Geometry check sheet. Reference: the model listing, model coordinates, mm. Face numbers are marked on the shaded views. Coordinates: 2 decimals unless noted, no trailing zeros. Loops run counter-clockwise (first coordinate to the right, second up) from the corner with the lowest first, then second, coordinate; pieces in that order, holes last. Notation, with made-up numbers: (-33.75, 7.5) - (19.25, 7.5) arc R24 ccw to (19.25, 19.5) - close; hole circle Ø7 at (18, 33). An arc over 180 degrees is marked (long way). Write each question's results on one line, items separated by ' | '. Start each with the question number.
(1) Material ranges on probe 1 along X at (y, z) = (-23, 14.5); probe 2 along Y at (x, z) = (5, 4.75); probe 3 along X at (y, z) = (-15.5, 5), recorded low to high.
(2) Sectioned sample at C-C (x = 5). Enter the section's corners in (y, z), plus the area to 3 significant figures.
(3) Sectioned sample at A-A (x = 0). Enter the section's corners in (y, z).
(4) Sectioned sample at B-B (y = -33). Enter the section's corners in (x, z), plus the area to 3 significant figures.
(5) Go/stop test with flat-tipped pins: pin 1 Ø5 at (x, z) = (11.5, 4.5) entering from -Y; pin 2 Ø5 at (y, z) = (-3.5, 8.5) entering from -X; pin 3 Ø10 at (y, z) = (-1, 16.5) entering from +X; pin 4 Ø8 at (y, z) = (-27, 15.5) entering from -X. Record where each tip stops, or that it passes through.
(6) Mould release check, pull along Y, two halves, no side actions. Record for the marked faces 1 and 2: pulls with the +Y half, pulls with the -Y half, needs draft (parallel to the pull), parting line crosses it, or undercut.
from build123d import *

# Parameters (mm, degrees)
F1_DEPTH = 20
F2_R     = 1.59999


# Not quite as in the source:
# - a fillet or chamfer is up to 0.001 mm smaller than in the source, because OpenCascade refuses the exact size


with BuildPart() as f1:
    # F0 (on Top) → F1 (new body)
    with BuildSketch(Plane.XY):
        with BuildLine():
            ThreePointArc((6.05, 0), (5.4927369002, -2.5362060928), (3.9236061669, -4.6051943115))
            Line((3.9236061669, -4.6051943115), (-1.4025425598, -9.1430506051))
            ThreePointArc((-1.4025425598, -9.1430506051), (-0.799716174, -9.2153651062), (-0.1934443699, -9.2479770369))
            ThreePointArc((-0.1934443699, -9.2479770369), (1.8772842283, -8.6355074503), (4.015398341, -8.3330112302))
            ThreePointArc((4.015398341, -8.3330112302), (5.0486509404, -7.7507176237), (5.9989019907, -7.0409995672))
            ThreePointArc((5.9989019907, -7.0409995672), (8.3979861697, -3.8776704725), (9.25, 0))
            ThreePointArc((9.25, 0), (-1.6062456434, 9.1094717154), (-8.6921567423, -3.1636863258))
            Line((-8.6921567423, -3.1636863258), (-5.6851403558, -2.0692218671))
            ThreePointArc((-5.6851403558, -2.0692218671), (-1.0505714749, 5.9580869057), (6.05, 0))
        make_face()
        with BuildLine():
            ThreePointArc((4.015398341, -8.3330112302), (1.9649742101, -9.0388813663), (-0.1934443699, -9.2479770369))
            ThreePointArc((-0.1934443699, -9.2479770369), (-2.4740598171, -10.3418630972), (-4.5333901906, -11.8105196067))
            ThreePointArc((-4.5333901906, -11.8105196067), (-1.1623519941, -36.3459888319), (19.7, -23))
            ThreePointArc((19.7, -23), (19.0087472673, -18.5452272785), (17, -14.5094169811))
            Line((17, -14.5094169811), (14.387755102, -16.3577071621))
            ThreePointArc((14.387755102, -16.3577071621), (15.9592240527, -19.5149737213), (16.5, -23))
            ThreePointArc((16.5, -23), (0.1791123856, -33.4407395624), (-2.4580943668, -14.2463248624))
            Line((-2.4580943668, -14.2463248624), (4.5116719892, -8.3081132677))
            ThreePointArc((4.5116719892, -8.3081132677), (4.2634299557, -8.3184651834), (4.015398341, -8.3330112302))
        make_face()
        with BuildLine():
            ThreePointArc((-0.1934443699, -9.2479770369), (-0.799716174, -9.2153651062), (-1.4025425598, -9.1430506051))
            Line((-1.4025425598, -9.1430506051), (-4.5333901906, -11.8105196067))
            ThreePointArc((-4.5333901906, -11.8105196067), (-2.4740598171, -10.3418630972), (-0.1934443699, -9.2479770369))
        make_face()
        with BuildLine():
            ThreePointArc((4.015398341, -8.3330112302), (1.8772842283, -8.6355074503), (-0.1934443699, -9.2479770369))
            ThreePointArc((-0.1934443699, -9.2479770369), (1.9649742101, -9.0388813663), (4.015398341, -8.3330112302))
        make_face()
        with BuildLine():
            ThreePointArc((5.9989019907, -7.0409995672), (5.0486509404, -7.7507176237), (4.015398341, -8.3330112302))
            ThreePointArc((4.015398341, -8.3330112302), (4.2634299557, -8.3184651834), (4.5116719892, -8.3081132677))
            Line((4.5116719892, -8.3081132677), (5.9989019907, -7.0409995672))
        make_face()
    extrude(amount=F1_DEPTH)

    # F2 (radius 1.6 in the source; OpenCascade refuses exactly that, so slightly less here)
    f2_edges = [f1.edges().sort_by_distance(p)[0] for p in [
        (17, -14.509417, 10),
        (14.387755, -16.357707, 10),
        (-8.692157, -3.163686, 10),
        (-5.68514, -2.069222, 10),
    ]]
    fillet(f2_edges, radius=F2_R)


solid = f1.part
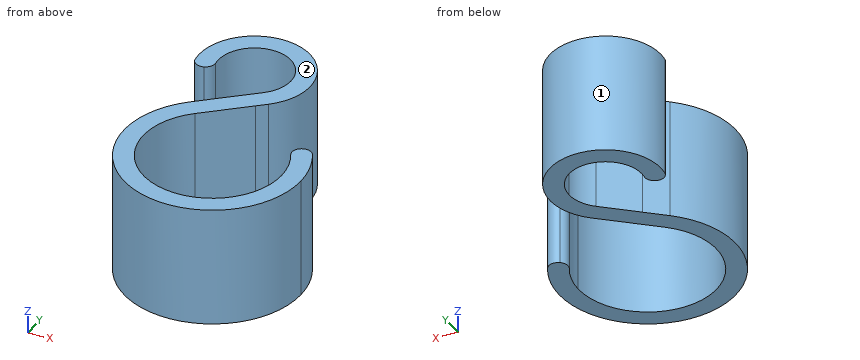
Outcome:
1) probe 1: x = -9.7 to -6.5, 16.5 to 19.7 | probe 2: y = -37.7 to -34.5, -7.89 to -3.41, 3.41 to 7.78 | probe 3: x = -7.64 to -3.72, 15.6 to 17.48
2) outline: (-37.7, 0) - (-34.5, 0) - (-34.5, 20) - (-37.7, 20) - close; (-7.89, 0) - (-3.41, 0) - (-3.41, 20) - (-7.89, 20) - close; (3.41, 0) - (7.78, 0) - (7.78, 20) - (3.41, 20) - close | area: 241 mm2
3) outline: (-36.82, 0) - (-33.36, 0) - (-33.36, 20) - (-36.82, 20) - close; (-12.15, 0) - (-7.95, 0) - (-7.95, 20) - (-12.15, 20) - close; (6.05, 0) - (9.25, 0) - (9.25, 20) - (6.05, 20) - close
4) outline: (-5.77, 0) - (-0.68, 0) - (-0.68, 20) - (-5.77, 20) - close; (10.68, 0) - (15.77, 0) - (15.77, 20) - (10.68, 20) - close | area: 204 mm2
5) pin 1: stops at y = -37.15 | pin 2: stops at x = -9.2 | pin 3: stops at x = 9.25 | pin 4: stops at x = -9.7
6) face 1: undercut | face 2: needs draft
